The listing builds one solid part. Answer for the finished solid, in the listing's coordinates (mm). A direction names the side the tool comes from. Coordinates: 2 decimals unless noted, no trailing zeros. Order: outer loops, then holes, each group sorted by start corner. A loop starts at its lowest first (then second) coordinate and runs counter-clockwise, first axis right, second up. Notation, with made-up numbers: (-22.5, -35) -> (22.5, -35) arc R17 cw to (22.5, -16) -> close; hole circle Ø11 at (61, 6). An arc over 180 degrees is marked (long way). Return JSON: item names as keys, results as strings.
Autodesk Inventor part; units mm, degrees
ref_plane "YZ Plane" through (0, 0, 0) normal (1, 0, 0) x (0, 1, 0)
ref_plane "XZ Plane" through (0, 0, 0) normal (0, 1, 0) x (-1, 0, 0)
ref_plane "XY Plane" through (0, 0, 0) normal (0, 0, 1) x (1, 0, 0)
sketch "Sketch1" plane through (0, 0, 0) normal (0, 0, 1) x (1, 0, 0)
  line L0 (0, 0) -> (16, 0)
  line L1 (16, 0) -> (16, 16)
  line L2 (16, 16) -> (0, 16)
  line L3 (0, 16) -> (0, 0)
  circle A0 centre (8, 8) radius 6
  dimension "d0" = 16
  dimension "d1" = 8
  dimension "d2" = 8
  dimension "d3" = 12
extrude "Extrusion2" add sketch "Sketch1" along normal blind 0.7 contours A0
sketch "Sketch3" plane through (8, 8, 0.7) normal (0, 0, 1) x (1, 0, 0)
  circle A0 centre (0, 0) radius 5
  circle A1 centre (0, 0) radius 6
  point P0 (-8, -8)
  dimension "d10" = 10
extrude "Extrusion3" add sketch "Sketch3" along normal blind 4 contours A0
fillet "Fillet1" radius 1 1 edges at (3, 8, 4.7)
fillet "Fillet1" radius 0.5 1 edges at (3, 8, 0.7)
properties part number "Foot"
Item 1: Flat-ended cylindrical pins translate along their axes: pin 1 (1 mm diameter, centred on y = 6, z = 3.5, fed in from +X); pin 2 (1.5 mm diameter, centred on x = 6.5, z = 4, fed in from -Y); pin 3 (1.5 mm diameter, centred on x = 5.5, z = 2.5, fed in from +Y). Find the tip coordinate at first contact, or state that the pin passes through.
Answer list:
{"pin 1": "x = 12.77", "pin 2": "y = 3.06", "pin 3": "y = 12.68"}
Item 2: The part is cut by section D-D on z = 2.5. Determine the outline of the cut face in (x, y).
Answer list:
{"outline": "circle Ø10 at (8, 8)"}
Item 3: Find the intervals of material crossed by probe 1 along Y at (x, z) = (5, 1.65); probe 2 along Y at (x, z) = (4.5, 1.3); probe 3 along X at (y, z) = (3.75, 0.3), in increasing order.
Answer list:
{"probe 1": "4 to 12", "probe 2": "4.43 to 11.57", "probe 3": "3.76 to 12.24"}
Item 4: The part is cut by section C-C on z = 0.4. Determine the outline of the cut face in (x, y).
Answer list:
{"outline": "circle Ø12 at (8, 8)"}
Item 5: Which of the six approach directions +Z, -Z, +X, -X, +Y, -Y give full straight-line access (tool end or side, diameter ignored) to faces 1 (the flat face through (8, 8, 0)), 2 (the cylindrical face through (12.77, 6.5, 2.43))?
Answer list:
{"face 1": "-Z, +X, -X, +Y, -Y", "face 2": "+Z"}
Item 6: The part is cut by section A-A on x = 8. Determine the outline of the cut face in (y, z), plus the area to 3 significant figures.
Answer list:
{"outline": "(2, 0) -> (14, 0) -> (14, 0.7) -> (13.5, 0.7) arc R0.5 cw to (13, 1.2) -> (13, 3.7) arc R1 ccw to (12, 4.7) -> (4, 4.7) arc R1 ccw to (3, 3.7) -> (3, 1.2) arc R0.5 cw to (2.5, 0.7) -> (2, 0.7) -> close", "area": "48.1 mm2"}
